Part print with two shaded views. Sizes in mm from the minimum x, y, z corner. Round coordinates to 2 decimals unless told otherwise and drop trailing zeros. Write each loop counter-clockwise with the first axis right and the second up, starting at its lowest first coordinate (ties: lowest second). Pieces come first, ordered by that corner, then holes. Notation, with made-up numbers: (45, -0.5) -> (92, -0.5) arc R32 cw to (92, 29.5) -> close; hole circle Ø3 at (-11.5, -31). An arc over 180 degrees is marked (long way). Answer in a Markdown table with one row per item.
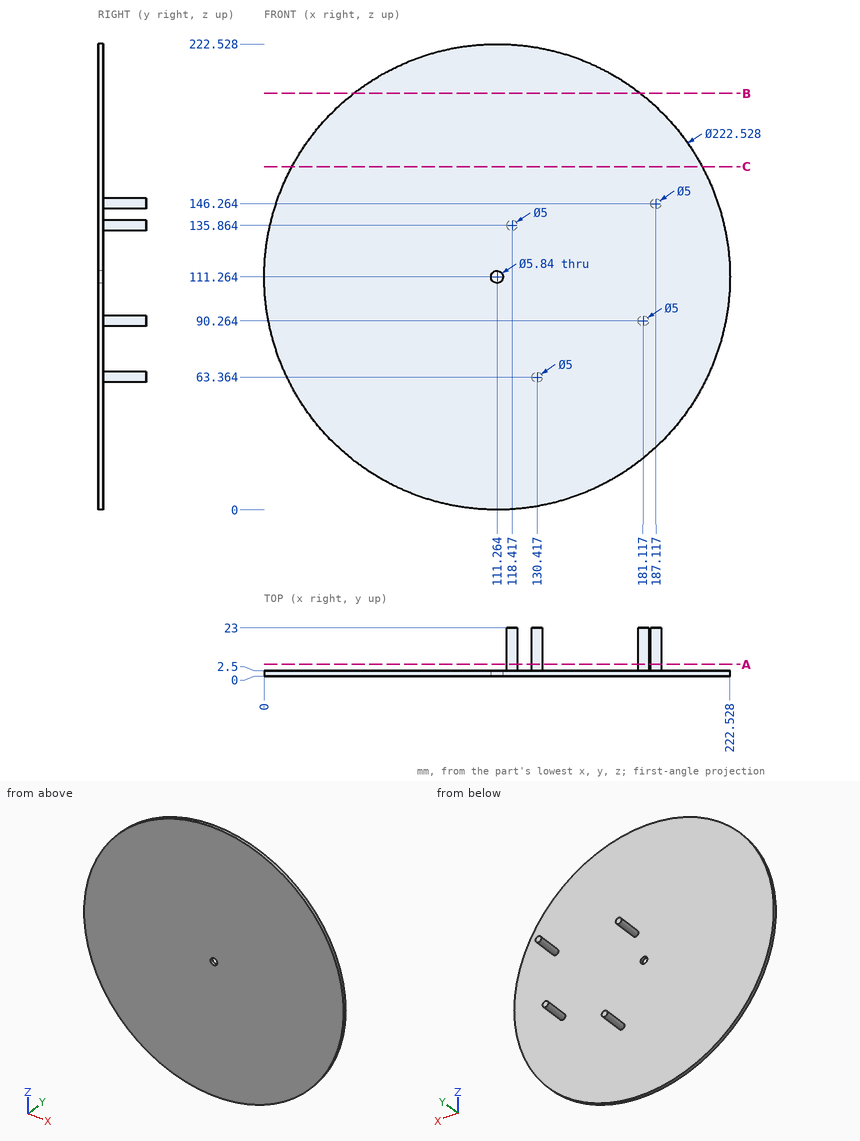
Q1. Wall check: line 1 (Y direction, x = 90.5, z = 144.5); line 2 (X direction, y = 3.25, z = 63); line 3 (Z direction, x = 132, y = 18.25). Give the ranges that are in metal, low to high. Write a range as [from, to].
A:
| item | result |
|---|---|
| line 1 | [0, 2.5] |
| line 2 | [127.94, 132.89] |
| line 3 | [61.43, 65.3] |
Q2. Saw through at C-C on z = 164. Write the cut outline in (x, y).
A:
| item | result |
|---|---|
| outline | (13.29, 0) -> (209.24, 0) -> (209.24, 2.5) -> (13.29, 2.5) -> close |
Q3. Drop flat-ended pins along their axis: P1, Ø5, axis at x = 135, z = 122, coming from the +Y side; P2, Ø4, axis at y = 4, z = 186.5, coming from the -X side; P3, Ø10, axis at y = 13, z = 130.5, coming from the +X side. Give the stop position or say it passes through.
A:
| item | result |
|---|---|
| P1 | y = 2.5 |
| P2 | x = 28.1 |
| P3 | x = 120.89 |
Q4. Saw through at A-A on y = 5.5. Write the cut outline in (x, z) (1 decimal).
A:
| item | result |
|---|---|
| outline | circle Ø5 at (118.4, 135.9); circle Ø5 at (130.4, 63.4); circle Ø5 at (181.1, 90.3); circle Ø5 at (187.1, 146.3) |
Q5. Saw through at B-B on z = 199. Write the cut outline in (x, y), plus the area to 3 significant figures.
A:
| item | result |
|---|---|
| outline | (42.84, 0) -> (179.69, 0) -> (179.69, 2.5) -> (42.84, 2.5) -> close |
| area | 342 mm² |
